Geometry check sheet. Reference: the model listing, model coordinates, mm. A direction names the side the tool comes from. Round coordinates to 2 decimals unless told otherwise and drop trailing zeros. Write each loop counter-clockwise with the first axis right and the second up, starting at its lowest first coordinate (ties: lowest second). Pieces come first, ordered by that corner, then holes. Notation, with made-up numbers: (-7.5, 2.5) - (-3.5, 2.5) arc R23 cw to (-3.5, 28.5) - close; hole circle Ø11 at (14, -10.75). An arc over 180 degrees is marked (long way). Return JSON: item names as keys, results as strings.
```python
from build123d import *

# Parameters (mm, degrees)
BOSS_EXTRUDE1_DEPTH = 2
BOSS_EXTRUDE3_DEPTH = 2


# Read off the part's stored shape, not the designer's step: Boss-Extrude3
with BuildPart() as part:
    # Sketch1 → Boss-Extrude1 (new body)
    with BuildSketch(Plane.XY):
        with BuildLine():
            Line((10.921700045, 15.820627971), (11.277420096, 13.949291525))
            Line((11.277420096, 13.949291525), (11.590342055, 15.907424067))
            ThreePointArc((11.590342055, 15.907424067), (11.725761981, 16.148644901), (11.985330235, 16.244302459))
            Line((11.985330235, 16.244302459), (14.707676179, 16.244302459))
            ThreePointArc((14.707676179, 16.244302459), (15.872864002, 15.546401169), (16.35465827, 14.27651804))
            Line((16.35465827, 14.27651804), (16.367622155, 13.819582081))
            ThreePointArc((16.367622155, 13.819582081), (15.803130226, 12.056353518), (14.259159222, 11.034698173))
            ThreePointArc((14.259159222, 11.034698173), (13.45100908, 10.884495001), (12.630428485, 10.836379176))
            Line((12.630428485, 10.836379176), (12.123518451, 10.838420989))
            Line((12.123518451, 10.838420989), (11.968610095, 9.869070376))
            Line((11.968610095, 9.869070376), (12.30473343, 7.884872777))
            ThreePointArc((12.30473343, 7.884872777), (12.19685885, 7.586331563), (11.905484198, 7.460376837))
            Line((11.905484198, 7.460376837), (10.999839261, 7.460376837))
            Line((10.999839261, 7.460376837), (10.724808345, 7.460376837))
            ThreePointArc((10.724808345, 7.460376837), (10.4163856, 7.605670319), (10.332021927, 7.935999785))
            Line((10.332021927, 7.935999785), (10.664596921, 9.663397929))
            Line((10.664596921, 9.663397929), (7.22360923, 9.783007686))
            Line((7.22360923, 9.783007686), (6.375331355, 7.946169859))
            ThreePointArc((6.375331355, 7.946169859), (6.218562023, 7.771225984), (5.990616105, 7.714457672))
            Line((5.990616105, 7.714457672), (5.298180624, 7.751850988))
            ThreePointArc((5.298180624, 7.751850988), (4.97142736, 7.954619126), (4.966617202, 8.339144126))
            Line((4.966617202, 8.339144126), (9.007156407, 15.933805165))
            ThreePointArc((9.007156407, 15.933805165), (9.1543162, 16.08882219), (9.36028944, 16.145930044))
            Line((9.36028944, 16.145930044), (10.528736663, 16.145930044))
            ThreePointArc((10.528736663, 16.145930044), (10.783806094, 16.054052723), (10.921700045, 15.820627971))
        make_face()
        with BuildLine():
            Line((12.232297108, 11.847227843), (12.862297108, 15.267227843))
            Line((12.862297108, 15.267227843), (13.989185775, 15.191954828))
            ThreePointArc((13.989185775, 15.191954828), (14.760146227, 14.789523159), (14.98451661, 13.949291525))
            Line((14.98451661, 13.949291525), (14.895254355, 13.372120047))
            ThreePointArc((14.895254355, 13.372120047), (14.287898045, 12.28062731), (13.116402, 11.847227843))
            Line((13.116402, 11.847227843), (12.232297108, 11.847227843))
        make_face(mode=Mode.SUBTRACT)
        Polygon((9.869863773, 14.885930044), (10.499863773, 10.745930044), (7.709863773, 10.835930044), align=None, mode=Mode.SUBTRACT)
    extrude(amount=BOSS_EXTRUDE1_DEPTH)

    # Boss-Extrude3 outline → Boss-Extrude3 (add)
    with BuildSketch(Plane.XY.offset(2)):
        with BuildLine():
            Line((10.528736641, 16.145925468), (9.36028944, 16.145930044))
            ThreePointArc((9.36028944, 16.145930044), (9.1543162, 16.08882219), (9.007156407, 15.933805165))
            Line((9.007156407, 15.933805165), (4.966617202, 8.339144126))
            ThreePointArc((4.966617202, 8.339144126), (4.97142736, 7.954619126), (5.298180624, 7.751850988))
            Line((5.298180624, 7.751850988), (5.990616105, 7.714457672))
            ThreePointArc((5.990616105, 7.714457672), (6.218562023, 7.771225984), (6.375331355, 7.946169859))
            Line((6.375331355, 7.946169859), (7.22360923, 9.783007686))
            Line((7.22360923, 9.783007686), (10.664596921, 9.663397929))
            Line((10.664596921, 9.663397929), (10.960889342, 7.797640802))
            ThreePointArc((10.960889342, 7.797640802), (11.096222191, 7.556161112), (11.355938946, 7.460376837))
            Line((11.355938946, 7.460376837), (11.905483631, 7.460416896))
            ThreePointArc((11.905483631, 7.460416896), (12.207123715, 7.604318029), (12.294240301, 7.926971058))
            Line((12.294240301, 7.926971058), (11.277420096, 13.949291525))
            Line((11.277420096, 13.949291525), (10.919712975, 15.821015565))
            ThreePointArc((10.919712975, 15.821015565), (10.782477337, 16.05356798), (10.528736641, 16.145925468))
        make_face()
        Polygon((10.499863773, 10.745930044), (7.709863773, 10.835930044), (9.869863773, 14.885930044), align=None, mode=Mode.SUBTRACT)
    extrude(amount=BOSS_EXTRUDE3_DEPTH)


solid = part.part
```
(1) Section check B-B, the plane x = 13.5. Enter the section's corners in (y, z), plus the area to 3 significant figures.
Response values:
{"outline": "(10.89, 0) - (11.89, 0) - (11.89, 2) - (10.89, 2) - close; (15.22, 0) - (16.24, 0) - (16.24, 2) - (15.22, 2) - close", "area": "4.04 mm^2"}
(2) Gauge pin test, flat ends, axial feed: pin 1 (1 mm diameter, centred on y = 12, z = 3, fed in from +X); pin 2 (0.9 mm diameter, centred on x = 9.5, z = 3, fed in from +Y); pin 3 (1.5 mm diameter, centred on x = 13, y = 12, fed in from +Z). Record the tip position at first contact, or that the pin passes through.
Response values:
{"pin 1": "stops at x = 11.69", "pin 2": "stops at y = 16.15", "pin 3": "stops at z = 2"}
(3) Access from +Z, -Z, +X, -X, +Y, -Y to the whole of each face (thin tool, end or side, straight path). Record for faces 1 (the face through (14.3, 12.29, 0.99)), 2 (the face through (10.81, 8.74, 2.99)), 3 (the face through (10, 16.146, 1)).
Response values:
{"face 1": "+Z, -Z", "face 2": "+Z, -Y", "face 3": "+Z, -Z, -X, +Y"}
(4) Section check A-A, the plane z = 0.5. Give the number of separate pieces and of enclosed holes in the cut face, plus the area to 3 significant figures.
Response values:
{"separate pieces": "1", "enclosed holes": "2", "area": "43.3 mm^2"}
(5) Section check C-C, the plane y = 13.25. Enter the section's corners in (x, z).
Response values:
{"outline": "(7.58, 0) - (9, 0) - (9, 4) - (7.58, 4) - close; (10.12, 0) - (12.49, 0) - (12.49, 2) - (11.4, 2) - (11.4, 4) - (10.12, 4) - close; (14.87, 0) - (16.33, 0) - (16.33, 2) - (14.87, 2) - close"}
(6) Material ranges on line 1 along X through (y, z) = (13, 1); line 2 along X through (y, z) = (12, 0.8); line 3 along X through (y, z) = (12.5, 2.85), recorded low to high. Write a range as [from, to].
Response values:
{"line 1": "x = [7.45, 8.86], [10.16, 12.44], [14.8, 16.27]", "line 2": "x = [6.91, 8.33], [10.31, 12.26], [13.84, 15.76]", "line 3": "x = [7.18, 8.6], [10.23, 11.52]"}
(7) Section check D-D, the plane z = 3.65. Enter the section's corners in (x, y), plus the area to 3 significant figures.
Response values:
{"outline": "(4.97, 8.34) arc R0.4 ccw to (5.3, 7.75) - (5.99, 7.71) arc R0.4 ccw to (6.38, 7.95) - (7.22, 9.78) - (10.66, 9.66) - (10.96, 7.8) arc R0.4 ccw to (11.36, 7.46) - (11.91, 7.46) arc R0.4 ccw to (12.29, 7.93) - (11.28, 13.95) - (10.92, 15.82) arc R0.4 ccw to (10.53, 16.15) - (9.36, 16.15) arc R0.4 ccw to (9.01, 15.93) - close; hole (7.71, 10.84) - (10.5, 10.75) - (9.87, 14.89) - close", "area": "26.1 mm^2"}
(8) Release check for a two-part mould opening along Y. For faces 4 (the face through (12.134, 8.891, 0.986)), 5 (the face through (13.42, 15.23, 0.99)), 6 (the face through (10.7, 8.2, 2)), 7 (the face through (7.015, 12.19, 1.972)) record: pulls with the +Y half, pulls with the -Y half, needs draft (parallel to the pull), parting line crosses it, or undercut.
Response values:
{"face 4": "undercut", "face 5": "undercut", "face 6": "needs draft", "face 7": "pulls with the +Y half"}
